For this review, take the finished solid that the model builds, in its own axes (mm). A direction names the side the tool comes from. Coordinates: 2 decimals unless noted, no trailing zeros. Order: outer loops, then holes, each group sorted by start corner. A loop starts at its lowest first (then second) coordinate and runs counter-clockwise, first axis right, second up. Notation, with made-up numbers: M 32,65.5 L 75,65.5 A28 cw 75,83.5 Z; hole C 18,-7 d8. An arc over 180 degrees is marked long. Use CSV: the item, a comma, the result in double quotes.
```python
from build123d import *

# Parameters (mm, degrees)
SKETCH1_W            = 25.4
SKETCH1_H            = 12.7
BOSS_EXTRUDE1_DEPTH  = 2.54
SKETCH1_3_R          = 1.9812
BOSS_EXTRUDE2_DEPTH  = 1.1938
LPATTERN1_COUNT      = 4
LPATTERN1_PITCH      = 6.35
LPATTERN1_COUNT_DIR2 = 2
LPATTERN1_PITCH_DIR2 = 6.35
SHELL1_T             = -1.1938
SKETCH2_R            = 2.5019
SKETCH2_R_2          = 1.9812
BOSS_EXTRUDE3_DEPTH  = 1.3462
LPATTERN2_COUNT      = 3
LPATTERN2_PITCH      = 6.35
FILLET1_R            = 1.1938


with BuildPart() as part:
    # Sketch1 → Boss-Extrude1 (new body)
    with BuildSketch(Plane(origin=(0, 0, 0), x_dir=(1, 0, 0), z_dir=(0, 1, 0))):
        with Locations((12.7, 6.35)):
            Rectangle(SKETCH1_W, SKETCH1_H)
    extrude(amount=-BOSS_EXTRUDE1_DEPTH)

    # Sketch1<3> → Boss-Extrude2 (add)
    with BuildSketch(Plane(origin=(0, 0, 0), x_dir=(1, 0, 0), z_dir=(0, 1, 0))):
        with Locations((3.175, 9.525)):
            Circle(SKETCH1_3_R)
    boss_extrude2 = extrude(amount=BOSS_EXTRUDE2_DEPTH)

    # LPattern1: Boss-Extrude2 4 × 2
    with Locations(*[(i * LPATTERN1_PITCH, 0, j * LPATTERN1_PITCH_DIR2) for i in range(LPATTERN1_COUNT) for j in range(LPATTERN1_COUNT_DIR2) if (i, j) != (0, 0)]):
        add(boss_extrude2)

    # Shell1
    shell1_openings = [part.faces().sort_by_distance(p)[0] for p in [
        (12.7, -2.54, -6.35),
    ]]
    offset(amount=SHELL1_T, openings=shell1_openings, kind=Kind.INTERSECTION)

    # Sketch2 → Boss-Extrude3 (add)
    with BuildSketch(Plane.XZ.offset(1.1938)):
        with Locations((6.337930238, -6.35)):
            Circle(SKETCH2_R)
        with Locations((6.337930238, -6.35)):
            Circle(SKETCH2_R_2, mode=Mode.SUBTRACT)
    boss_extrude3 = extrude(amount=BOSS_EXTRUDE3_DEPTH)

    # LPattern2: Boss-Extrude3 ×3
    with Locations(*[(i * LPATTERN2_PITCH, 0, 0) for i in range(1, LPATTERN2_COUNT)]):
        add(boss_extrude3)

    # Fillet1
    fillet1_edges = [part.edges().sort_by_distance(p)[0] for p in [
        (1.1938, -1.8669, -1.1938),
        (1.1938, -1.8669, -11.5062),
        (24.2062, -1.8669, -11.5062),
        (24.2062, -1.8669, -1.1938),
    ]]
    fillet(fillet1_edges, radius=FILLET1_R)


solid = part.part
```
Item 1: For faces 4 (the face through (22, 1.194, -3)), 5 (the face through (16, 0, -10)), 6 (the face through (24.055, 0.589, -2.416)), list the 3-axis set-ups (+Z, -Z, +X, -X, +Y, -Y) from which the entire face can be reached by the end or side of a thin tool; tool diameter is ignored.
Solutions:
face 4,"+Z, -Z, +X, -X, +Y"
face 5,"-Y"
face 6,"+Y"
Item 2: Clearance check with flat-ended pins moving along their axes: pin 1 Ø1.3 at (x, z) = (3.175, -3.175) entering from -Y; pin 2 Ø3 at (x, z) = (12.5, -5) entering from -Y; pin 3 Ø1.7 at (x, z) = (22, -9.5) entering from -Y. State where each tip first meets the part, or that it passes through.
Solutions:
pin 1,"y = 0"
pin 2,"y = -2.54"
pin 3,"y = -1.19"
Item 3: Draft analysis for pull direction Z (two halves, no side actions). For faces 1 (the face through (22, 1.194, -10)), 2 (the face through (13, -1, 0)), 3 (the face through (19, -1.194, -6)), state which applies: released by +Z, released by -Z, zero draft, split by the parting line, or undercut.
Solutions:
face 1,"zero draft"
face 2,"released by +Z"
face 3,"undercut"
Item 4: Add section D-D on x = 16.25. State the section outline as (y, z) points, and give its area (3 significant figures).
Solutions:
outline,"M -2.54,-12.7 L 0,-12.7 L 0,-11.47 L 1.19,-11.47 L 1.19,-7.58 L 0,-7.58 L 0,-5.12 L 1.19,-5.12 L 1.19,-1.23 L 0,-1.23 L 0,0 L -2.54,0 L -2.54,-1.19 L -1.19,-1.19 L -1.19,-2.48 L 0,-2.48 L 0,-3.87 L -1.19,-3.87 L -1.19,-8.83 L 0,-8.83 L 0,-10.22 L -1.19,-10.22 L -1.19,-11.51 L -2.54,-11.51 Z"
area,"24.4 mm^2"
Item 5: Add section C-C on x = 1.5. State the section outline as (y, z) points.
Solutions:
outline,"M -2.54,-12.7 L 0,-12.7 L 0,-10.58 L 1.19,-10.58 L 1.19,-8.47 L 0,-8.47 L 0,-4.23 L 1.19,-4.23 L 1.19,-2.12 L 0,-2.12 L 0,0 L -2.54,0 L -2.54,-1.59 L -1.19,-1.59 L -1.19,-11.11 L -2.54,-11.11 Z"
Item 6: To check wall thickness, follow line 1 along Z through (x, y) = (3.75, -0.2); line 2 along X through (y, z) = (0.9, -10.25); line 3 along Z through (x, y) = (12.5, -1.75). State the ranges of each line that lie inside material, in increasing order. Write a range as [from, to].
Solutions:
line 1,"[-12.7, -10.06], [-8.99, -3.71], [-2.64, 0]"
line 2,"[1.33, 5.02], [7.68, 11.37], [14.03, 17.72], [20.38, 24.07]"
line 3,"[-12.7, -11.51], [-8.84, -8.32], [-4.38, -3.86], [-1.19, 0]"
Item 7: Add section B-B on x = 6.75. State the section outline as (y, z) points.
Solutions:
outline,"M -2.54,-12.7 L 0,-12.7 L 0,0 L -2.54,0 L -2.54,-1.19 L -1.19,-1.19 L -1.19,-3.88 L -2.54,-3.88 L -2.54,-4.41 L -1.19,-4.41 L -1.19,-8.29 L -2.54,-8.29 L -2.54,-8.82 L -1.19,-8.82 L -1.19,-11.51 L -2.54,-11.51 Z"
